Work out the finished part from the listing and answer in its coordinate system (mm). Coordinates: 2 decimals unless noted, no trailing zeros. Order: outer loops, then holes, each group sorted by start corner. A loop starts at its lowest first (then second) coordinate and runs counter-clockwise, first axis right, second up. Notation, with made-up numbers: (88.25, -22.5) - (128.25, -22.5) arc R34 cw to (128.25, 8.5) - close; hole circle Ø11 at (-12, 70). An arc over 180 degrees is marked (long way). Answer as a JSON object with one key per item and string values. Group by question number.
1) Section B-B (z = -101.5) is taken. Count the separate pieces of the cut face and the enclosed holes in it, plus the area to 3 significant figures.
2) Each of these flat-tipped pins is pushed along its axis until it touches: P1, Ø2, axis at y = 118.5, z = 21, coming from the +X side; P2, Ø1.1, axis at x = -471.5, y = 36.5, coming from the -Z side; P3, Ø3, axis at x = 248.5, y = 70.5, coming from the -Z side. Where does it stop, or does it pass through?
3) Section A-A (x = -644.5) is taken. Give the vertices of the cut face in (y, z), plus the area to 3 significant figures.
4) Find the intervals of material crossed by line 1 along Y through (x, z) = (-181.5, 152); line 2 along Z through (x, y) = (-79, 29.5); line 3 along X through (y, z) = (60, -163), in increasing order.
5) Section C-C (y = 77.5) is taken. Give the vertices of the cut face in (x, z), plus the area to 3 significant figures.
from build123d import *

# Parameters (mm, degrees)
SKETCH1_W           = 1920
SKETCH1_H           = 440
BOSS_EXTRUDE1_DEPTH = 40
SKETCH4_W           = 1754
SKETCH4_H           = 320
BOSS_EXTRUDE2_DEPTH = 80
SKETCH5_W           = 1754
SKETCH5_H           = 320
SKETCH5_W_2         = 1714
SKETCH5_H_2         = 280
CUT_EXTRUDE1_DEPTH  = 3
SKETCH6_W           = 1754
SKETCH6_H           = 320
SKETCH6_W_2         = 1748
SKETCH6_H_2         = 314
CUT_EXTRUDE2_DEPTH  = 20
SKETCH7_W           = 40
SKETCH7_H           = 280
CUT_EXTRUDE3_DEPTH  = 4
SKETCH8_W           = 1920
SKETCH8_H           = 440
SKETCH8_W_2         = 1880
SKETCH8_H_2         = 400
CUT_EXTRUDE4_DEPTH  = 3
SKETCH9_W           = 1920
SKETCH9_H           = 440
SKETCH9_W_2         = 1914
SKETCH9_H_2         = 434
CUT_EXTRUDE5_DEPTH  = 20
SKETCH10_W          = 40
SKETCH10_H          = 400
CUT_EXTRUDE9_DEPTH  = 4


with BuildPart() as part:
    # Sketch1 → Boss-Extrude1 (new body)
    with BuildSketch(Plane(origin=(0, 0, 0), x_dir=(1, 0, 0), z_dir=(0, 1, 0))):
        with Locations((0, 10)):
            Rectangle(SKETCH1_W, SKETCH1_H)
    extrude(amount=BOSS_EXTRUDE1_DEPTH)

    # Sketch4 → Boss-Extrude2 (add)
    with BuildSketch(Plane(origin=(0, 40, 0), x_dir=(1, 0, 0), z_dir=(0, 1, 0))):
        with Locations((0, 30)):
            Rectangle(SKETCH4_W, SKETCH4_H)
    extrude(amount=BOSS_EXTRUDE2_DEPTH)

    # Sketch5 → Cut-Extrude1 (cut)
    with BuildSketch(Plane(origin=(0, 120, 0), x_dir=(1, 0, 0), z_dir=(0, 1, 0))):
        with Locations((0, 30)):
            Rectangle(SKETCH5_W, SKETCH5_H)
        with Locations((0, 30)):
            Rectangle(SKETCH5_W_2, SKETCH5_H_2, mode=Mode.SUBTRACT)
    extrude(amount=-CUT_EXTRUDE1_DEPTH, mode=Mode.SUBTRACT)

    # Sketch6 → Cut-Extrude2 (cut)
    with BuildSketch(Plane(origin=(0, 120, 0), x_dir=(1, 0, 0), z_dir=(0, 1, 0))):
        with Locations((0, 30)):
            Rectangle(SKETCH6_W, SKETCH6_H)
        with Locations((0, 30)):
            Rectangle(SKETCH6_W_2, SKETCH6_H_2, mode=Mode.SUBTRACT)
    extrude(amount=-CUT_EXTRUDE2_DEPTH, mode=Mode.SUBTRACT)

    # Sketch7 → Cut-Extrude3 (cut)
    with BuildSketch(Plane(origin=(0, 120, 0), x_dir=(1, 0, 0), z_dir=(0, 1, 0))):
        with Locations((480, 30)):
            Rectangle(SKETCH7_W, SKETCH7_H)
        with Locations((-480, 30)):
            Rectangle(SKETCH7_W, SKETCH7_H)
    extrude(amount=-CUT_EXTRUDE3_DEPTH, mode=Mode.SUBTRACT)

    # Sketch8 → Cut-Extrude4 (cut)
    with BuildSketch(Plane(origin=(0, 40, 0), x_dir=(1, 0, 0), z_dir=(0, 1, 0))):
        with Locations((0, 10)):
            Rectangle(SKETCH8_W, SKETCH8_H)
        with Locations((0, 10)):
            Rectangle(SKETCH8_W_2, SKETCH8_H_2, mode=Mode.SUBTRACT)
    extrude(amount=-CUT_EXTRUDE4_DEPTH, mode=Mode.SUBTRACT)

    # Sketch9 → Cut-Extrude5 (cut)
    with BuildSketch(Plane(origin=(0, 40, 0), x_dir=(1, 0, 0), z_dir=(0, 1, 0))):
        with Locations((0, 10)):
            Rectangle(SKETCH9_W, SKETCH9_H)
        with Locations((0, 10)):
            Rectangle(SKETCH9_W_2, SKETCH9_H_2, mode=Mode.SUBTRACT)
    extrude(amount=-CUT_EXTRUDE5_DEPTH, mode=Mode.SUBTRACT)

    # Sketch10 → Cut-Extrude9 (cut)
    with BuildSketch(Plane(origin=(0, 40, 0), x_dir=(1, 0, 0), z_dir=(0, 1, 0))):
        with Locations((-480, 10)):
            Rectangle(SKETCH10_W, SKETCH10_H)
        with Locations((480, 10)):
            Rectangle(SKETCH10_W, SKETCH10_H)
    extrude(amount=-CUT_EXTRUDE9_DEPTH, mode=Mode.SUBTRACT)


solid = part.part
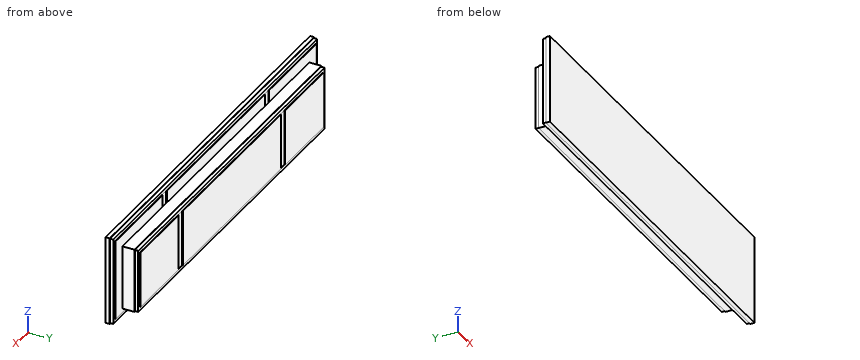
Report:
{
 "1": {"separate pieces": "1", "enclosed holes": "2", "area": "216,000 mm²"},
 "2": {"P1": "stops at x = 857", "P2": "stops at z = -227", "P3": "stops at z = -190"},
 "3": {"outline": "(0, -230) - (20, -230) - (20, -227) - (37, -227) - (37, -210) - (40, -210) - (40, -190) - (100, -190) - (100, -187) - (117, -187) - (117, -170) - (120, -170) - (120, 110) - (117, 110) - (117, 127) - (100, 127) - (100, 130) - (40, 130) - (40, 190) - (37, 190) - (37, 207) - (20, 207) - (20, 210) - (0, 210) - close", "area": "42,800 mm²"},
 "4": {"line 1": "y = 0 to 40", "line 2": "z = -227 to 207", "line 3": "x = -877 to 877"},
 "5": {"outline": "(-877, -190) - (877, -190) - (877, 130) - (-877, 130) - close", "area": "561,000 mm²"}
}
